```python
from build123d import *
from build123d.topology import SkipClean

# Parameters (mm, degrees)
SKETCH_1_R          = 35
SKETCH_1_R_2        = 30
SKETCH_1_R_3        = 1.5
SKETCH_1_R_4        = 26
SKETCH_1_R_5        = 20
SKETCH_1_R_6        = 15
SKETCH_1_R_7        = 12.5
EXTRUDE_1_DEPTH     = 5
EXTRUDE_START       = 10
SKETCH_2_R          = 30
SKETCH_2_R_2        = 26
SKETCH_2_R_3        = 1.5
SKETCH_2_R_4        = 20
SKETCH_2_R_5        = 15
EXTRUDE_2_DEPTH     = 10
SKETCH_3_R          = 4
SKETCH_3_R_2        = 1.5
CUT_EXTRUDE_1_DEPTH = 10


with BuildPart() as part:
    # 草图1 → 凸台-拉伸1 (new body)
    # profile 1 of 6: a face of its own
    with BuildSketch(Plane.XY):
        Circle(SKETCH_1_R)
        Circle(SKETCH_1_R_2, mode=Mode.SUBTRACT)
    # profile 2 of 6: a face of its own
    with BuildSketch(Plane.XY):
        Circle(SKETCH_1_R_2)
        with Locations((-28, 0)):
            Circle(SKETCH_1_R_3, mode=Mode.SUBTRACT)
        with Locations((0, -28)):
            Circle(SKETCH_1_R_3, mode=Mode.SUBTRACT)
        with Locations((28, 0)):
            Circle(SKETCH_1_R_3, mode=Mode.SUBTRACT)
        with Locations((0, 28)):
            Circle(SKETCH_1_R_3, mode=Mode.SUBTRACT)
        Circle(SKETCH_1_R_4, mode=Mode.SUBTRACT)
    # profile 3 of 6: a face of its own
    with BuildSketch(Plane.XY):
        Circle(SKETCH_1_R_4)
        Circle(SKETCH_1_R_5, mode=Mode.SUBTRACT)
    # profile 4 of 6: a face of its own
    with BuildSketch(Plane.XY):
        Circle(SKETCH_1_R_5)
        with Locations((-17.5, 0)):
            Circle(SKETCH_1_R_3, mode=Mode.SUBTRACT)
        with Locations((0, -17.5)):
            Circle(SKETCH_1_R_3, mode=Mode.SUBTRACT)
        with Locations((17.5, 0)):
            Circle(SKETCH_1_R_3, mode=Mode.SUBTRACT)
        with Locations((0, 17.5)):
            Circle(SKETCH_1_R_3, mode=Mode.SUBTRACT)
        Circle(SKETCH_1_R_6, mode=Mode.SUBTRACT)
    # profile 5 of 6: a face of its own
    with BuildSketch(Plane.XY):
        Circle(SKETCH_1_R_6)
        Circle(SKETCH_1_R_7, mode=Mode.SUBTRACT)
    # profile 6 of 6: a face of its own
    with BuildSketch(Plane.XY):
        Circle(SKETCH_1_R_7)
    extrude(amount=EXTRUDE_1_DEPTH)

    # 草图2 → 凸台-拉伸2 (add)
    # profile 1 of 2: a face of its own
    with SkipClean():  # the faces are left unmerged after this step: merging them gives an invalid solid
        with BuildSketch(Plane(origin=(0, 0, 0), x_dir=(-1, 0, 0), z_dir=(0, 0, -1)).offset(EXTRUDE_START)):
            with Locations(Location((0, 0, 0), (0, 0, 180))):
                Circle(SKETCH_2_R)
            Circle(SKETCH_2_R_2, mode=Mode.SUBTRACT)
            with Locations((0, -28)):
                Circle(SKETCH_2_R_3, mode=Mode.SUBTRACT)
            with Locations((0, 28)):
                Circle(SKETCH_2_R_3, mode=Mode.SUBTRACT)
            with Locations((-28, 0)):
                Circle(SKETCH_2_R_3, mode=Mode.SUBTRACT)
            with Locations((28, 0)):
                Circle(SKETCH_2_R_3, mode=Mode.SUBTRACT)
        # profile 2 of 2: a face of its own
        with BuildSketch(Plane(origin=(0, 0, 0), x_dir=(-1, 0, 0), z_dir=(0, 0, -1)).offset(EXTRUDE_START)):
            with Locations(Location((0, 0, 0), (0, 0, 180))):
                Circle(SKETCH_2_R_4)
            Circle(SKETCH_2_R_5, mode=Mode.SUBTRACT)
            with Locations((17.5, 0)):
                Circle(SKETCH_2_R_3, mode=Mode.SUBTRACT)
            with Locations((-17.5, 0)):
                Circle(SKETCH_2_R_3, mode=Mode.SUBTRACT)
            with Locations((0, 17.5)):
                Circle(SKETCH_2_R_3, mode=Mode.SUBTRACT)
            with Locations((0, -17.5)):
                Circle(SKETCH_2_R_3, mode=Mode.SUBTRACT)
        extrude(amount=-EXTRUDE_2_DEPTH)

    # 草图3 → 切除-拉伸1 (cut)
    with SkipClean():  # the faces are left unmerged after this step: merging them gives an invalid solid
        with BuildSketch(Plane(origin=(0, 0, 0), x_dir=(-1, 0, 0), z_dir=(0, 0, -1))):
            with BuildLine():
                ThreePointArc((-3.5, 5), (-6.060660172, 6.060660172), (-5, 3.5))
                Line((-5, 3.5), (-5, 5))
                Line((-5, 5), (-3.5, 5))
            make_face()
            with BuildLine():
                Line((-5, 5), (-5, 3.5))
                ThreePointArc((-5, 3.5), (-3.939339828, 3.939339828), (-3.5, 5))
                Line((-3.5, 5), (-5, 5))
            make_face()
            Circle(SKETCH_3_R)
            with Locations((-5, -5)):
                Circle(SKETCH_3_R_2)
            with Locations((5, -5)):
                Circle(SKETCH_3_R_2)
            with Locations((5, 5)):
                Circle(SKETCH_3_R_2)
        extrude(amount=-CUT_EXTRUDE_1_DEPTH, mode=Mode.SUBTRACT)


solid = part.part
```
CAD build for the part. Positions are in the model's coordinates, mm. A direction names the side the tool comes from. Round coordinates to 2 decimals unless told otherwise and drop trailing zeros. Order: outer loops, then holes, each group sorted by start corner. A loop starts at its lowest first (then second) coordinate and runs counter-clockwise, first axis right, second up. Notation, with made-up numbers: (-31.5, 3) - (-5.5, 3) arc R27 cw to (-5.5, 25) - close; hole circle Ø11 at (77.25, 15.5). An arc over 180 degrees is marked (long way). Answer in a Markdown table with one row per item. Add a question column.
(1) Drop flat-ended pins along their axis: pin 1 Ø4 at (x, y) = (5, 5) entering from -Z; pin 2 Ø2 at (y, z) = (23, -4) entering from -X; pin 3 Ø2.5 at (x, y) = (-5, -5) entering from -Z; pin 4 Ø6 at (x, z) = (-2, 0) entering from +Y. Give the stop position or say it passes through.
(2) Mould opens along Y. For faces 3 (the face through (0, -7, 5)), 4 (the face through (16.128, -25.296, -5.07)), 5 (the face through (20.633, -15.821, -5.07)) say: +Y half, -Y half, draft (parallel to the pull), parting line (faces both ways), or undercut.
(3) Band-saw the part on D-D on y = -17.5. List the corners of the cut face in (x, z), and give its area (3 significant figures).
(4) Band-saw the part on A-A on z = -6. Count the separate pieces of the cut face and the enclosed holes in it, and give its area (3 significant figures).
(5) Probe L1, parallel to Y at x = 0, z = 1.15; L2, parallel to X at y = 10.5, z = -6.25; L3, parallel to Y at x = -8.5, z = -7. List the from-to ranges inside material, lowest first. Write a range as [from, to].
(6) 3-axis set-ups, long thin cutter, end or side, ignore diameter. For faces 1 (the face through (-25, 9, -10)), 2 (the face through (26, 16, 0)): which of +Z, -Z, +X, -X, +Y, -Y reach the whole face in a straight line?
Data:
| question | item | result |
|---|---|---|
| 1 | pin 1 | stops at z = 0 |
| 1 | pin 2 | stops at x = -20.4 |
| 1 | pin 3 | passes through |
| 1 | pin 4 | stops at y = 35 |
| 2 | face 3 | draft |
| 2 | face 4 | parting line |
| 2 | face 5 | undercut |
| 3 | outline | (-30.31, 0) - (-24.37, 0) - (-24.37, -10) - (-19.23, -10) - (-19.23, 0) - (-9.68, 0) - (-9.68, -10) - (-1.5, -10) - (-1.5, 5) - (-30.31, 5) - close; (1.5, -10) - (9.68, -10) - (9.68, 0) - (19.23, 0) - (19.23, -10) - (24.37, -10) - (24.37, 0) - (30.31, 0) - (30.31, 5) - (1.5, 5) - close |
| 3 | area | 555 mm^2 |
| 4 | separate pieces | 2 |
| 4 | enclosed holes | 10 |
| 4 | area | 1,200 mm^2 |
| 5 | L1 | y = [-35, -29.5], [-26.5, -19], [-16, -4], [4, 16], [19, 26.5], [29.5, 35] |
| 5 | L2 | x = [-28.1, -23.79], [-17.02, -10.71], [10.71, 17.02], [23.79, 28.1] |
| 5 | L3 | y = [-28.77, -24.57], [-18.1, -12.36], [12.36, 18.1], [24.57, 28.77] |
| 6 | face 1 | -Z, +X, -X, +Y, -Y |
| 6 | face 2 | -Z |
